Geometry: final body of the model. Coordinates: model frame, mm. Face numbers are marked on the shaded views. Coordinates: 2 decimals unless noted, no trailing zeros. Order: outer loops, then holes, each group sorted by start corner. A loop starts at its lowest first (then second) coordinate and runs counter-clockwise, first axis right, second up. Notation, with made-up numbers: (76, 20) -> (127, 20) arc R34 cw to (127, 55) -> close; hole circle Ø4 at (79, 27.5). An arc over 180 degrees is marked (long way). Answer in a Markdown table with one row per item. Add a question column.
1) Pull-direction query (Y, two-part tool) for the marked faces 1, 2 and 3; classes: +Y half, -Y half, draft (parallel to the pull), parting line (faces both ways), or undercut.
2) Section query C-C on z = 0.6. Return the cut outline in (x, y) (3 decimals).
3) Ray query, line 1 (Y direction, x = 0, z = 1.7) (3 decimals); line 2 (Z direction, x = 5, y = 9). Return the intervals inside material, ascending. Write a range as from..to.
4) Section query D-D on x = 11.5. Return the cut outline in (y, z).
5) Section query A-A on y = 0. Return the cut outline in (x, z) (3 decimals).
6) Contact query for a flat-ended pin moving along its axis: P1, Ø1.5, axis at x = 10, z = 1, coming from the -Y side. Output: stop coordinate, or through.
Autodesk Inventor part; units mm, degrees
ref_plane "YZ Plane" through (0, 0, 0) normal (1, 0, 0) x (0, 1, 0)
ref_plane "XZ Plane" through (0, 0, 0) normal (0, 1, 0) x (-1, 0, 0)
ref_plane "XY Plane" through (0, 0, 0) normal (0, 0, 1) x (1, 0, 0)
sketch "Sketch1" plane through (0, 0, 0) normal (0, 1, 0) x (-1, 0, 0)
  line L0 (4.5, 0) -> (4.5, 3)
  line L1 (4.5, 3) -> (6.5, 3)
  line L2 (6.5, 3) -> (7.5, 2)
  line L3 (7.5, 2) -> (14.875, 2)
  line L4 (14.875, 2) -> (14.875, 0)
  line L5 (14.875, 0) -> (4.5, 0)
  line L6 (0, 0) -> (0, 4.9053) construction
  dimension "d0" = 14.875
  dimension "d1" = 4.5
  dimension "d2" = 6.5
  dimension "d3" = 2
  dimension "d4" = 3
  dimension "d5" = 1
revolve "Revolution1" add sketch "Sketch1" angle 360 about axis through (0, 0, 0) along (0, 0, 1)
fillet "Fillet1" radius 1 2 edges at (7.5, 0, 2) (6.5, 0, 3)
properties part number "washer"
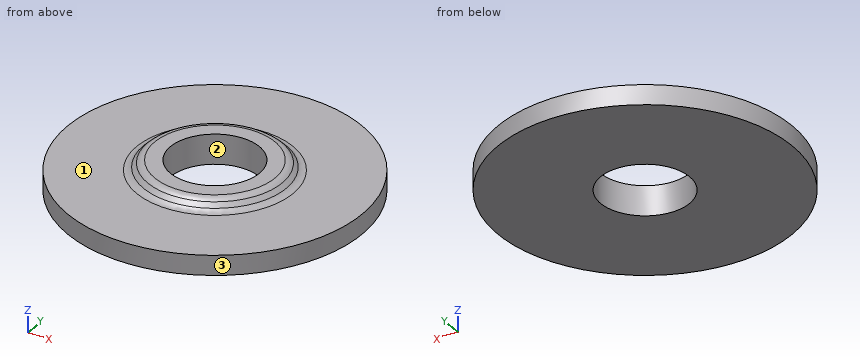
Result:
| question | item | result |
|---|---|---|
| 1 | face 1 | draft |
| 1 | face 2 | undercut |
| 1 | face 3 | parting line |
| 2 | outline | circle Ø29.75 at (0, 0); hole circle Ø9 at (0, 0) |
| 3 | line 1 | -14.875..-4.5, 4.5..14.875 |
| 3 | line 2 | 0..2 |
| 4 | outline | (-9.43, 0) -> (9.43, 0) -> (9.43, 2) -> (-9.43, 2) -> close |
| 5 | outline | (-14.875, 0) -> (-4.5, 0) -> (-4.5, 3) -> (-6.086, 3) arc R1 ccw to (-6.793, 2.707) -> (-7.207, 2.293) arc R1 cw to (-7.914, 2) -> (-14.875, 2) -> close; (4.5, 0) -> (14.875, 0) -> (14.875, 2) -> (7.914, 2) arc R1 cw to (7.207, 2.293) -> (6.793, 2.707) arc R1 ccw to (6.086, 3) -> (4.5, 3) -> close |
| 6 | P1 | y = -11.65 |
